Model file for the job. Use its own axes, mm. A direction names the side the tool comes from. Give positions to 0.01 mm unless a question says otherwise; leave off trailing zeros. Loops run counter-clockwise (first coordinate to the right, second up) from the corner with the lowest first, then second, coordinate; pieces in that order, holes last. Notation, with made-up numbers: M 65,11 L 119,11 A18 cw 119,39 Z; hole C 0,52.25 d7. An arc over 180 degrees is marked long. Answer in a Markdown table with one row per item.
```python
from build123d import *

# Parameters (mm, degrees)
PAD_DEPTH = 115


with BuildPart() as part:
    # Sketch → Pad (new body, symmetric)
    with BuildSketch(Plane.XZ):
        Polygon((0, 51), (0, 0), (51, 0), (51, 4), (4, 4), (4, 51), align=None)
    extrude(amount=PAD_DEPTH, both=True)


solid = part.part
```
Q1. Drop flat-ended pins along their axis: pin 1 (6 mm diameter, centred on x = 24.5, y = 46, fed in from +Z); pin 2 (14 mm diameter, centred on y = -32, z = 17, fed in from +X). Give the stop position or say it passes through.
Reported:
| item | result |
|---|---|
| pin 1 | z = 4 |
| pin 2 | x = 4 |
Q2. Saw through at A-A (y = -99.5). Give the cut face in (x, z).
Reported:
| item | result |
|---|---|
| outline | M 0,0 L 51,0 L 51,4 L 4,4 L 4,51 L 0,51 Z |
Q3. Probe probe 1 along X at (y, z) = (-105.5, 47.5). List the from-to ranges inside material, lowest first.
Reported:
| item | result |
|---|---|
| probe 1 | 0 to 4 |
Q4. Saw through at B-B (x = 12.5). Give the cut face in (y, z), and give its area (3 significant figures).
Reported:
| item | result |
|---|---|
| outline | M -115,0 L 115,0 L 115,4 L -115,4 Z |
| area | 920 mm² |
Q5. Saw through at C-C (z = 36). Give the cut face in (x, y).
Reported:
| item | result |
|---|---|
| outline | M 0,-115 L 4,-115 L 4,115 L 0,115 Z |
Q6. 3-axis set-ups, long thin cutter, end or side, ignore diameter. For faces 1 (the face through (25, -2, 0)), 2 (the face through (28, -2, 4)): which of +Z, -Z, +X, -X, +Y, -Y reach the whole face in a straight line?
Reported:
| item | result |
|---|---|
| face 1 | -Z, +X, -X, +Y, -Y |
| face 2 | +Z, +X, +Y, -Y |
